Here's how the part is built. I have some questions about the finished solid (model axes, mm). Face numbers are marked on the shaded views. Round coordinates to 2 decimals unless told otherwise and drop trailing zeros. Loops run counter-clockwise (first coordinate to the right, second up) from the corner with the lowest first, then second, coordinate; pieces in that order, holes last. Notation, with made-up numbers: M 69,42 L 101,42 A16 ccw 101,59 Z; hole C -6.75,-3.5 d9. An arc over 180 degrees is marked long. Put each result on its own line as item: value. Start each with the question number.
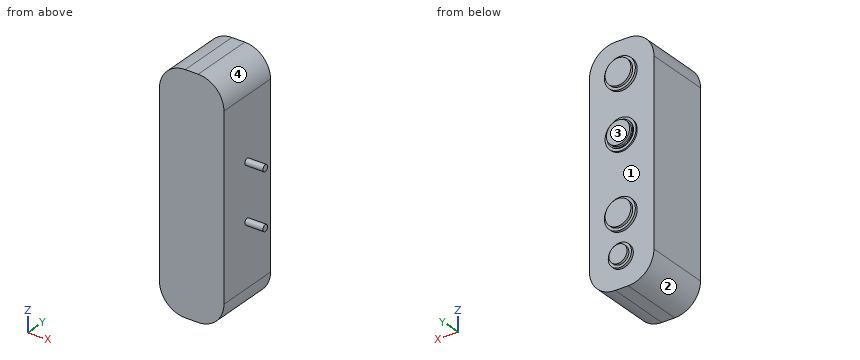
```python
from build123d import *

# Parameters (mm, degrees)
SKETCH1_W           = 25
SKETCH1_H           = 90
BOSS_EXTRUDE1_DEPTH = 25
SKETCH2_R           = 5
SKETCH2_R_2         = 3.5
SKETCH2_R_3         = 4.5
BOSS_EXTRUDE2_DEPTH = 2
SKETCH2_3_R         = 6
SKETCH2_3_R_2       = 4.5
SKETCH2_3_R_3       = 5
BOSS_EXTRUDE3_DEPTH = 1
SKETCH2_4_R         = 6
BOSS_EXTRUDE4_DEPTH = 0.6
FILLET1_R           = 10
SKETCH3_R           = 1.25
BOSS_EXTRUDE5_DEPTH = 7


with BuildPart() as part:
    # Sketch1 → Boss-Extrude1 (new body)
    with BuildSketch(Plane(origin=(0, 0, 0), x_dir=(1, 0, 0), z_dir=(0, 1, 0))):
        Rectangle(SKETCH1_W, SKETCH1_H)
    extrude(amount=BOSS_EXTRUDE1_DEPTH)

    # Sketch2 → Boss-Extrude2 (add)
    with BuildSketch(Plane(origin=(0, 25, 0), x_dir=(1, 0, 0), z_dir=(0, 1, 0))):
        with Locations((0, -32.5)):
            Circle(SKETCH2_R)
        with Locations((0, 18.5)):
            Circle(SKETCH2_R)
        with Locations((0, 33.5)):
            Circle(SKETCH2_R_2)
        with Locations((0, -10.5)):
            Circle(SKETCH2_R_3)
    extrude(amount=BOSS_EXTRUDE2_DEPTH)

    # Sketch2<3> → Boss-Extrude3 (add)
    with BuildSketch(Plane(origin=(0, 25, 0), x_dir=(1, 0, 0), z_dir=(0, 1, 0))):
        with Locations((0, -32.5)):
            Circle(SKETCH2_3_R)
        with Locations((0, 18.5)):
            Circle(SKETCH2_3_R)
        with Locations((0, 33.5)):
            Circle(SKETCH2_3_R_2)
        with Locations((0, -10.5)):
            Circle(SKETCH2_3_R_3)
    extrude(amount=BOSS_EXTRUDE3_DEPTH)

    # Sketch2<4> → Boss-Extrude4 (add)
    with BuildSketch(Plane(origin=(0, 25, 0), x_dir=(1, 0, 0), z_dir=(0, 1, 0))):
        with Locations((0, -10.5)):
            Circle(SKETCH2_4_R)
    extrude(amount=BOSS_EXTRUDE4_DEPTH)

    # Fillet1
    fillet1_edges = [part.edges().sort_by_distance(p)[0] for p in [
        (12.5, 12.5, 45),
        (-12.5, 12.5, 45),
        (-12.5, 12.5, -45),
        (12.5, 12.5, -45),
    ]]
    fillet(fillet1_edges, radius=FILLET1_R)

    # Sketch3 → Boss-Extrude5 (add)
    with BuildSketch(Plane(origin=(12.5, 0, 0), x_dir=(0, 0, -1), z_dir=(1, 0, 0))):
        with Locations((-10.86, 12.5)):
            Circle(SKETCH3_R)
        with Locations((10.86, 12.5)):
            Circle(SKETCH3_R)
    extrude(amount=BOSS_EXTRUDE5_DEPTH)


solid = part.part
```
1) Suppose I cut it at D-D (z = -33.5). Write out the boundary of the cut face in (x, y).
2) Suppose I cut it at B-B (x = 14.5). Write out the boundary of the cut face in (y, z), plus the area to 3 significant figures.
3) Suppose I cut it at A-A (z = -18.5). Write out the boundary of the cut face in (x, y).
4) If we mould it in two halves opening along Z, with no side actions, what happens to the marked faces 1, 2, 3 and 4? For each: pulls with the +Z half, pulls with the -Z half, needs draft (parallel to the pull), parting line crosses it, or undercut.
5) I'm going to push flat-ended pins straight in: P1, Ø2, axis at x = -5, y = 13.5, coming from the +Z side; P2, Ø1.5, axis at x = -8.5, y = 4.5, coming from the +Z side; P3, Ø5, axis at x = 8.5, y = 23, coming from the +Z side. Where does each tip first touch, or does it pass through?
6) If I drill on probe 1 along Y at (x, z) = (5.5, 9); probe 2 along Y at (x, z) = (-1.5, -5); probe 3 along X at (y, z) = (7.75, -16), over which ranges is the centre line in solid material (lowest first)? Write a range as from..to.
7) Suppose I cut it at C-C (y = 12.5). Write out the boundary of the cut face in (x, z), plus the area to 3 significant figures.
Results are:
1. outline: M -12.5,0 L 12.5,0 L 12.5,25 L 4.5,25 L 4.5,26 L 3.5,26 L 3.5,27 L -3.5,27 L -3.5,26 L -4.5,26 L -4.5,25 L -12.5,25 Z
2. outline: C 12.5,-10.86 d2.5; C 12.5,10.86 d2.5
2. area: 9.82 mm²
3. outline: M -12.5,0 L 12.5,0 L 12.5,25 L 6,25 L 6,26 L 5,26 L 5,27 L -5,27 L -5,26 L -6,26 L -6,25 L -12.5,25 Z
4. face 1: undercut
4. face 2: pulls with the -Z half
4. face 3: needs draft
4. face 4: pulls with the +Z half
5. P1: z = 44.89
5. P2: z = 43.51
5. P3: z = 44.37
6. probe 1: 0..25.6
6. probe 2: 0..25
6. probe 3: -12.5..12.5
7. outline: M -12.5,-35 A10 ccw -2.5,-45 L 2.5,-45 A10 ccw 12.5,-35 L 12.5,-12.11 L 19.5,-12.11 L 19.5,-9.61 L 12.5,-9.61 L 12.5,9.61 L 19.5,9.61 L 19.5,12.11 L 12.5,12.11 L 12.5,35 A10 ccw 2.5,45 L -2.5,45 A10 ccw -12.5,35 Z
7. area: 2,200 mm²
